from build123d import *

# Parameters (mm, degrees)
F0_W     = 48.5
F0_H     = 47.25
F0_W_2   = 40.5
F0_H_2   = 39.25
F0_W_3   = 36.5
F0_H_3   = 35.25
F1_DEPTH = 2
F2_DEPTH = 3.2


with BuildPart() as f1:
    # F0 (on Top) → F1 (new body)
    with BuildSketch(Plane.XY):
        Rectangle(F0_W, F0_H)
        Rectangle(F0_W_2, F0_H_2, mode=Mode.SUBTRACT)
        Rectangle(F0_W_2, F0_H_2)
        Rectangle(F0_W_3, F0_H_3, mode=Mode.SUBTRACT)
        Rectangle(F0_W_3, F0_H_3)
    extrude(amount=F1_DEPTH)

    # F0 (on Top) → F2 (join)
    with BuildSketch(Plane.XY):
        Rectangle(F0_W_2, F0_H_2)
        Rectangle(F0_W_3, F0_H_3, mode=Mode.SUBTRACT)
    extrude(amount=F2_DEPTH)


solid = f1.part
Read the model definition and answer for the solid it produces. Units are mm, in the model's axes. A direction names the side the tool comes from. Round coordinates to 2 decimals unless told otherwise and drop trailing zeros. Write each loop counter-clockwise with the first axis right and the second up, starting at its lowest first coordinate (ties: lowest second). Pieces come first, ordered by that corner, then holes.
1. The part is cut by section C-C, the plane x = 19.5. Determine the outline of the cut face in (y, z) (3 decimals), then the cut area to 3 significant figures.
2. Determine the mould class of faces 5 (the face through (0, -19.625, 3)), 6 (the face through (0, 19.625, 3)), 7 (the face through (0, 0, 2)) for opening direction Y: pulls with the +Y half, pulls with the -Y half, needs draft (parallel to the pull), parting line crosses it, or undercut.
3. Straight lines are drawn through the part: L1, parallel to X at y = 9, z = 2.45; L2, parallel to Y at x = 15.5, z = 2.85 (3 decimals); L3, parallel to Z at x = 16.5, y = 2. For each, find the intervals that lie inside material, in ascending order.
4. The part is cut by section A-A, the plane z = 2.65. Determine the outline of the cut face in (x, y) (3 decimals), then the cut area to 3 significant figures.
5. The part is cut by section B-B, the plane y = -18.5. Determine the outline of the cut face in (x, z), then the cut area to 3 significant figures.
6. Which of the six approach directions +Z, -Z, +X, -X, +Y, -Y give full straight-line access (tool end or side, diameter ignored) to faces 1 (the face through (0, -23.625, 1)), 2 (the face through (20.25, 0, 3)), 3 (the face through (-20.25, 0, 3)), 4 (the face through (-18.25, 0, 3))?
7. The part is cut by section D-D, the plane y = -11. Determine the outline of the cut face in (x, z).
8. Given pin 1 Ø0.6 at (y, z) = (-3, 2.5) entering from -X; pin 2 Ø1.3 at (y, z) = (-1, 3) entering from +X; pin 3 Ø10 at (x, y) = (4, -5.5) entering from +Z, each flat-ended and moving along its own axis, determine where each tip first touches the part or whether it passes through.
Values:
1. outline: (-23.625, 0) - (23.625, 0) - (23.625, 2) - (19.625, 2) - (19.625, 3.2) - (-19.625, 3.2) - (-19.625, 2) - (-23.625, 2) - close
1. area: 142 mm2
2. face 5: pulls with the -Y half
2. face 6: pulls with the +Y half
2. face 7: undercut
3. L1: x = -20.25 to -18.25, 18.25 to 20.25
3. L2: y = -19.625 to -17.625, 17.625 to 19.625
3. L3: z = 0 to 2
4. outline: (-20.25, -19.625) - (20.25, -19.625) - (20.25, 19.625) - (-20.25, 19.625) - close; hole (-18.25, -17.625) - (18.25, -17.625) - (18.25, 17.625) - (-18.25, 17.625) - close
4. area: 303 mm2
5. outline: (-24.25, 0) - (24.25, 0) - (24.25, 2) - (20.25, 2) - (20.25, 3.2) - (-20.25, 3.2) - (-20.25, 2) - (-24.25, 2) - close
5. area: 146 mm2
6. face 1: +Z, -Z, +X, -X, -Y
6. face 2: +Z, +X, +Y, -Y
6. face 3: +Z, -X, +Y, -Y
6. face 4: +Z
7. outline: (-24.25, 0) - (24.25, 0) - (24.25, 2) - (20.25, 2) - (20.25, 3.2) - (18.25, 3.2) - (18.25, 2) - (-18.25, 2) - (-18.25, 3.2) - (-20.25, 3.2) - (-20.25, 2) - (-24.25, 2) - close
8. pin 1: stops at x = -20.25
8. pin 2: stops at x = 20.25
8. pin 3: stops at z = 2
